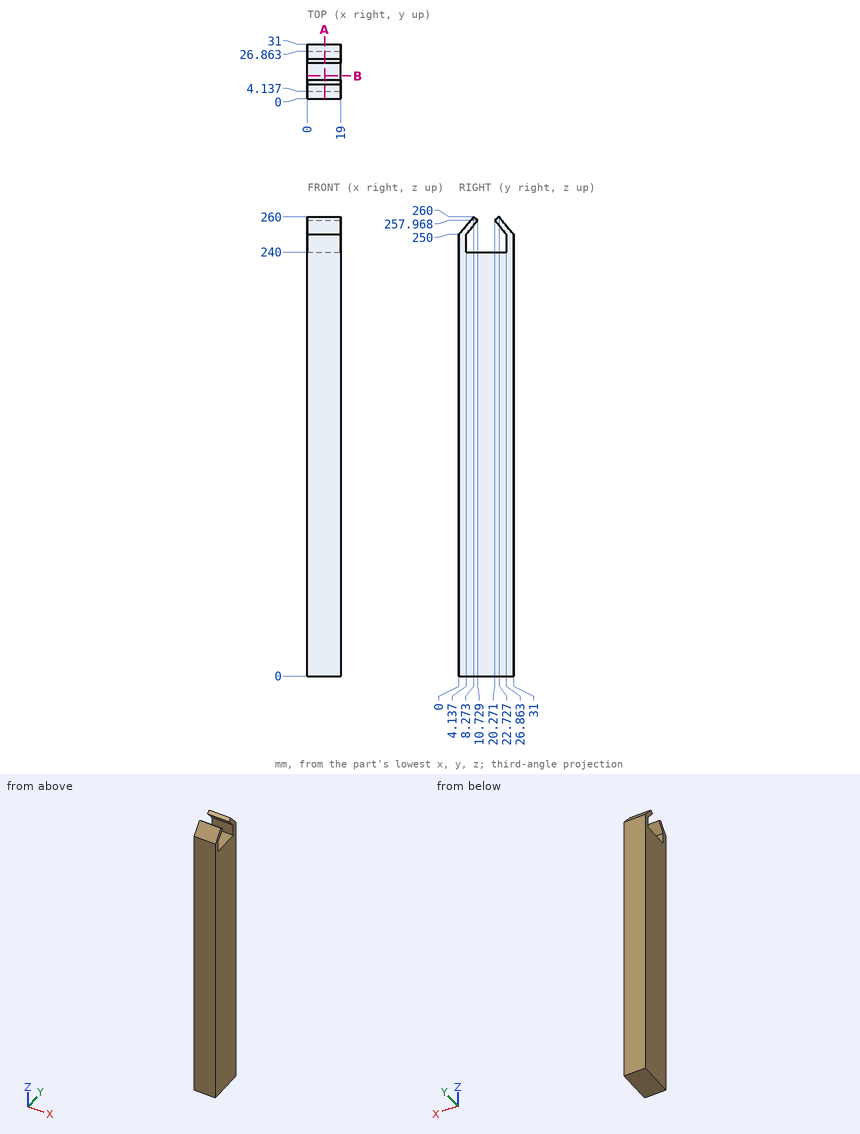
Job drawing, mm, ordinate dimensions from the low corner. One solid piece. Round coordinates to 2 decimals unless told otherwise and drop trailing zeros. Write each loop counter-clockwise with the first axis right and the second up, starting at its lowest first coordinate (ties: lowest second). Pieces come first, ordered by that corner, then holes. Notation, with made-up numbers: (-32.75, 52.5) -> (-12.75, 52.5) arc R3 cw to (-12.75, 57.5) -> close; hole circle Ø6 at (61, 0). An arc over 180 degrees is marked (long way). Answer as CSV lines item,"result".
1. Slice it at A-A, the plane x = 9.75. List the corners of the cut face in (y, z), plus the area to 3 significant figures.
Resolved:
outline,"(0, 0) -> (31, 0) -> (31, 250) -> (22.73, 260) -> (20.27, 257.97) -> (26.86, 250) -> (26.86, 240) -> (4.14, 240) -> (4.14, 250) -> (10.73, 257.97) -> (8.27, 260) -> (0, 250) -> close"
area,"7,600 mm²"
2. Slice it at B-B, the plane y = 13. List the corners of the cut face in (x, z), plus the area to 3 significant figures.
Resolved:
outline,"(0, 0) -> (19, 0) -> (19, 240) -> (0, 240) -> close"
area,"4,560 mm²"
3. Pin check, flat tips, straight feed: pin 1 Ø8 at (x, y) = (5, 13.5) entering from +Z (1 decimal); pin 2 Ø5 at (x, y) = (8, 18) entering from +Z. Stop position of each tip, or through.
Resolved:
pin 1,"z = 259"
pin 2,"z = 258.16"
4. Drill centre lines: line 1 (Z direction, x = 1, y = 8); line 2 (Z direction, x = 14.5, y = 14); line 3 (Z direction, x = 2.25, y = 10.5) (1 decimal). Where is each one in solid material? Low to high.
Resolved:
line 1,"0 to 240, 254.67 to 259.67"
line 2,"0 to 240"
line 3,"0 to 240, 257.7 to 258.2"
